Read the model definition and answer for the solid it produces. Units are mm, in the model's axes. Give positions to 0.01 mm unless a question says otherwise; leave off trailing zeros. Write each loop counter-clockwise with the first axis right and the second up, starting at its lowest first coordinate (ties: lowest second). Pieces come first, ordered by that corner, then holes. Notation, with made-up numbers: M -17,-36.75 L -6,-36.75 A36 cw -6,-0.75 Z; hole C -27.5,39 d11. An arc over 180 degrees is marked long. Put each result on its own line as item: value.
from build123d import *

# Parameters (mm, degrees)
F0_W     = 25
F0_H     = 40
F1_DEPTH = 3
F2_R     = 5


with BuildPart() as f1:
    # F0 (on Top) → F1 (new body)
    with BuildSketch(Plane.XY):
        Polygon((56.1464983402, 0), (-38.8535016598, 0), (-38.8535016598, -25), (81.1464983402, -25), (81.1464983402, 0), align=None)
        with BuildLine():
            ThreePointArc((-25.8535016598, -15.5), (-28.8535016598, -12.5), (-25.8535016598, -9.5))
            Line((-25.8535016598, -9.5), (10.752664879, -9.5))
            ThreePointArc((10.752664879, -9.5), (12.8739852225, -10.3786796564), (13.752664879, -12.5))
            ThreePointArc((13.752664879, -12.5), (12.8739852225, -14.6213203436), (10.752664879, -15.5))
            Line((10.752664879, -15.5), (-25.8535016598, -15.5))
        make_face(mode=Mode.SUBTRACT)
        with Locations((68.6464983402, 20)):
            Rectangle(F0_W, F0_H)
        with BuildLine():
            ThreePointArc((65.6464983402, 28), (68.6464983402, 31), (71.6464983402, 28))
            Line((71.6464983402, 28), (71.6464983402, 4.4783727005))
            ThreePointArc((71.6464983402, 4.4783727005), (68.6464983402, 1.4783727005), (65.6464983402, 4.4783727005))
            Line((65.6464983402, 4.4783727005), (65.6464983402, 28))
        make_face(mode=Mode.SUBTRACT)
    extrude(amount=F1_DEPTH)

    # F2
    f2_edges = [f1.edges().sort_by_distance(p)[0] for p in [
        (-38.853502, -25, 1.5),
        (81.146498, -25, 1.5),
        (-38.853502, 0, 1.5),
        (81.146498, 40, 1.5),
        (56.146498, 40, 1.5),
        (56.146498, 0, 1.5),
    ]]
    fillet(f2_edges, radius=F2_R)


solid = f1.part
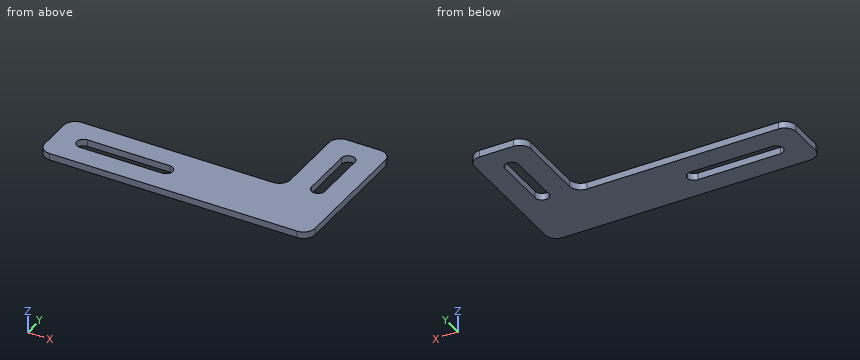
(1) Given pin 1 Ø1.5 at (x, z) = (16.5, 1.5) entering from +Y; pin 2 Ø0.9 at (y, z) = (22, 2) entering from -X; pin 3 Ø8 at (x, y) = (-13, -8.5) entering from -Z, each flat-ended and moving along its own axis, determine where each tip first touches the part or whether it passes through.
Result:
pin 1: stops at y = 0
pin 2: stops at x = 56.15
pin 3: stops at z = 0
(2) Section B-B on z = 0.7 is taken. Determine the outline of the cut face in (x, y).
Result:
outline: M -38.85,-20 A5 ccw -33.85,-25 L 76.15,-25 A5 ccw 81.15,-20 L 81.15,35 A5 ccw 76.15,40 L 61.15,40 A5 ccw 56.15,35 L 56.15,5 A5 cw 51.15,0 L -33.85,0 A5 ccw -38.85,-5 Z; hole M -25.85,-15.5 L 10.75,-15.5 A3 ccw 10.75,-9.5 L -25.85,-9.5 A3 ccw Z; hole M 65.65,4.48 A3 ccw 71.65,4.48 L 71.65,28 A3 ccw 65.65,28 Z
(3) Section D-D on x = 36 is taken. Determine the outline of the cut face in (y, z).
Result:
outline: M -25,0 L 0,0 L 0,3 L -25,3 Z
(4) Section C-C on y = 16 is taken. Determine the outline of the cut face in (x, z).
Result:
outline: M 56.15,0 L 65.65,0 L 65.65,3 L 56.15,3 Z; M 71.65,0 L 81.15,0 L 81.15,3 L 71.65,3 Z
(5) Section A-A on x = -14.5 is taken. Determine the outline of the cut face in (y, z), and give its area (3 significant figures).
Result:
outline: M -25,0 L -15.5,0 L -15.5,3 L -25,3 Z; M -9.5,0 L 0,0 L 0,3 L -9.5,3 Z
area: 57.0 mm²
(6) Straight lines are drawn through the part: line 1 along X through (y, z) = (5.5, 2.8); line 2 along Y through (x, z) = (2, 0.65); line 3 along X through (y, z) = (-12.5, 2.5). For each, find the intervals that lie inside material, in ascending order. Write a range as from..to.
Result:
line 1: x = 56.15..65.65, 71.65..81.15
line 2: y = -25..-15.5, -9.5..0
line 3: x = -38.85..-28.85, 13.75..81.15
